```python
from build123d import *

# Parameters (mm, degrees)
SKETCH1_R                = 5.60705
BOSS_EXTRUDE1_DEPTH      = 1.778
SKETCH2_R                = 10.16
BOSS_EXTRUDE2_DEPTH      = 4.318
SKETCH3_R                = 1.143
CUT_EXTRUDE1_DEPTH       = 3.318
SKETCH4_R                = 5.5626
BOSS_EXTRUDE3_DEPTH      = 3.0099
BOSS_EXTRUDE4_DEPTH      = 5.78485
FILLET1_R                = 2
FILLET2_R                = 2
SKETCH6_W                = 8.0772
SKETCH6_H                = 4.0386
CUT_EXTRUDE2_DEPTH       = 2.6924
CHAMFER1_SIZE            = 2.6924
CHAMFER1_OF_MIRROR2_SIZE = 2.6924
FILLET3_R                = 2
BOSS_EXTRUDE5_DEPTH      = 12.7
SKETCH8_R                = 2.48285
BOSS_EXTRUDE6_DEPTH      = 25.4


with BuildPart() as part:
    # Sketch1 → Boss-Extrude1 (new body)
    with BuildSketch(Plane(origin=(0, 0, 0), x_dir=(1, 0, 0), z_dir=(0, 1, 0))):
        with Locations(Location((0, 0, 0), (0, 0, 270))):
            Circle(SKETCH1_R)
    extrude(amount=-BOSS_EXTRUDE1_DEPTH)

    # Sketch2 → Boss-Extrude2 (add)
    with BuildSketch(Plane.XZ.offset(1.778)):
        with Locations(Location((0, 0, 0), (0, 0, 270))):
            Circle(SKETCH2_R)
    extrude(amount=BOSS_EXTRUDE2_DEPTH)

    # Sketch3 → Cut-Extrude1 (cut)
    with BuildSketch(Plane(origin=(0, -1.778, 0), x_dir=(1, 0, 0), z_dir=(0, 1, 0))):
        with Locations(Location((7.4, 0, 0), (0, 0, 270))):
            Circle(SKETCH3_R)
    cut_extrude1 = extrude(amount=-CUT_EXTRUDE1_DEPTH, mode=Mode.SUBTRACT)

    # Mirror1: Cut-Extrude1 across plane
    add(cut_extrude1.mirror(Plane(origin=(0, 0, 0), x_dir=(0, 0, 1), z_dir=(1, 0, 0))), mode=Mode.SUBTRACT)

    # Sketch4 → Boss-Extrude3 (add)
    with BuildSketch(Plane.XZ.offset(6.096)):
        with Locations(Location((0, 0, 0), (0, 0, 270))):
            Circle(SKETCH4_R)
    extrude(amount=BOSS_EXTRUDE3_DEPTH)

    # Sketch5 → Boss-Extrude4 (add, symmetric)
    with BuildSketch(Plane(origin=(0, 0, 0), x_dir=(0, 0, -1), z_dir=(1, 0, 0))):
        Polygon((-8.5344, -9.1059), (8.7757, -9.1059), (8.7757, -10.0203), (11.8237, -10.0203), (11.8237, -16.51), (-5.7912, -16.51), (-11.0236, -11.7983), (-11.0236, -10.0203), (-8.5344, -10.0203), align=None)
    extrude(amount=BOSS_EXTRUDE4_DEPTH, both=True)

    # Fillet1
    fillet1_edges = [part.edges().sort_by_distance(p)[0] for p in [
        (-5.78485, -9.5631, 8.5344),
        (-5.78485, -9.5631, -8.7757),
        (5.78485, -9.5631, 8.5344),
        (5.78485, -9.5631, -8.7757),
    ]]
    fillet(fillet1_edges, radius=FILLET1_R)

    # Fillet2
    fillet2_edges = [part.edges().sort_by_distance(p)[0] for p in [
        (-5.78485, -10.9093, 11.0236),
        (5.78485, -10.9093, 11.0236),
    ]]
    fillet(fillet2_edges, radius=FILLET2_R)

    # Sketch6 → Cut-Extrude2 (cut)
    with BuildSketch(Plane(origin=(5.78485, 0, 0), x_dir=(0, 0, -1), z_dir=(1, 0, 0))):
        with Locations((7.7851, -14.4907)):
            Rectangle(SKETCH6_W, SKETCH6_H)
    cut_extrude2 = extrude(amount=-CUT_EXTRUDE2_DEPTH, mode=Mode.SUBTRACT)

    # Chamfer1
    chamfer1_edges = [part.edges().sort_by_distance(p)[0] for p in [
        (3.09245, -14.4907, -3.7465),
    ]]
    chamfer(chamfer1_edges, length=CHAMFER1_SIZE - 0.0001)  # a hair under: the kernel refuses the full size

    # Mirror2: Cut-Extrude2 across plane
    add(cut_extrude2.mirror(Plane(origin=(0, 0, 0), x_dir=(0, 0, 1), z_dir=(1, 0, 0))), mode=Mode.SUBTRACT)

    # Chamfer1 of Mirror2
    chamfer1_of_mirror2_edges = [part.edges().sort_by_distance(p)[0] for p in [
        (-3.09245, -14.4907, -3.7465),
    ]]
    chamfer(chamfer1_of_mirror2_edges, length=CHAMFER1_OF_MIRROR2_SIZE - 0.0001)  # a hair under: the kernel refuses the full size

    # Fillet3
    fillet3_edges = [part.edges().sort_by_distance(p)[0] for p in [
        (-5.78485, -11.24585, -11.8237),
        (5.78485, -11.24585, -11.8237),
    ]]
    fillet(fillet3_edges, radius=FILLET3_R)

    # Sketch7 → Boss-Extrude5 (add)
    with BuildSketch(Plane(origin=(0, 0, -11.8237), x_dir=(-1, 0, 0), z_dir=(0, 0, -1))):
        Polygon((1.529978213, -15.681103357), (3.059956427, -13.031103357), (1.529978213, -10.381103357), (-1.529978213, -10.381103357), (-3.059956427, -13.031103357), (-1.529978213, -15.681103357), align=None)
    extrude(amount=BOSS_EXTRUDE5_DEPTH)

    # Sketch8 → Boss-Extrude6 (add)
    with BuildSketch(Plane(origin=(0, 0, -24.5237), x_dir=(-1, 0, 0), z_dir=(0, 0, -1))):
        with Locations((0, -13.007748328)):
            Circle(SKETCH8_R)
    extrude(amount=BOSS_EXTRUDE6_DEPTH)


solid = part.part
```
The model under review builds one solid part; all positions refer to its coordinate system, in mm. A direction names the side the tool comes from. Round coordinates to 2 decimals unless told otherwise and drop trailing zeros. Loops run counter-clockwise (first coordinate to the right, second up) from the corner with the lowest first, then second, coordinate; pieces in that order, holes last. Notation, with made-up numbers: (1, 57.5) - (40, 57.5) arc R34 ccw to (40, 96.5) - close; hole circle Ø10 at (38, -12.5). An arc over 180 degrees is marked (long way). Use a Markdown table: item, result. Add a question column.
Q1. The part is to be moulded in two halves that separate along Y. For faces 1 (the face through (-2.306, -11.725, -18.085)), 2 (the face through (-4, -12.471, -9)), 3 (the face through (-4.4, -6.096, -4.4)), 4 (the face through (-5.215, -11.263, -11.222)), say which applies: pulls with the +Y half, pulls with the -Y half, needs draft (parallel to the pull), parting line crosses it, or undercut.
Q2. Insertion check: pin 1 Ø2.5 at (x, z) = (0.5, -21) entering from +Y; pin 2 Ø3 at (x, y) = (3.5, -5.5) entering from +Z; pin 3 Ø3 at (x, z) = (5, -30.5) entering from -Y; pin 4 Ø2.5 at (x, z) = (0.5, -9) entering from +Y. Each pin has a flat end and moves straight along its axis. Give the tip position at first contact, or say it passes through.
Q3. Add section B-B (y = -4). State the section outline as (x, z) points, plus the area to 3 significant figures.
Q4. Add section A-A (z = 0). State the section outline as (x, y) points, plus the area to 3 significant figures.
Q5. Machinability: for faces 5 (the face through (-5.785, -13, 2)), 6 (the face through (4, -12.471, -9)), 7 (the face through (0, -15.681, -18)), 8 (the face through (5.785, -13, 2)), 9 (the face through (4.73, -0.88, 3.01)), which of the approach directions +Z, -Z, +X, -X, +Y, -Y give a long, thin tool a straight path to every point of the face, cutting with its end or side? Answer none if there is none.
Q6. For probe 1 along X at (y, z) = (-3.55, 0); probe 2 along Y at (x, z) = (5.5, 5); probe 3 along Z at (x, y) = (-7.4, -4.25), list the stretches that pass through material, from the lowest coordinate up.
Q7. Add section D-D (x = -8). State the section outline as (y, z) points, plus the area to 3 significant figures.
Worked answers:
| question | item | result |
|---|---|---|
| 1 | face 1 | pulls with the +Y half |
| 1 | face 2 | pulls with the -Y half |
| 1 | face 3 | undercut |
| 1 | face 4 | needs draft |
| 2 | pin 1 | y = -10.38 |
| 2 | pin 2 | z = 9.96 |
| 2 | pin 3 | through |
| 2 | pin 4 | y = -1.78 |
| 3 | outline | circle Ø20.32 at (0, 0); hole circle Ø2.29 at (-7.4, 0); hole circle Ø2.29 at (7.4, 0) |
| 3 | area | 316 mm² |
| 4 | outline | (-10.16, -6.1) - (-5.56, -6.1) - (-5.56, -9.11) - (-5.78, -9.11) - (-5.78, -16.51) - (5.78, -16.51) - (5.78, -9.11) - (5.56, -9.11) - (5.56, -6.1) - (10.16, -6.1) - (10.16, -1.78) - (8.54, -1.78) - (8.54, -5.1) - (6.26, -5.1) - (6.26, -1.78) - (5.61, -1.78) - (5.61, 0) - (-5.61, 0) - (-5.61, -1.78) - (-6.26, -1.78) - (-6.26, -5.1) - (-8.54, -5.1) - (-8.54, -1.78) - (-10.16, -1.78) - close |
| 4 | area | 212 mm² |
| 5 | face 5 | +Z, -Z, -X, -Y |
| 5 | face 6 | -Z, +X, -Y |
| 5 | face 7 | -Z, +X, -X, -Y |
| 5 | face 8 | +Z, -Z, +X, -Y |
| 5 | face 9 | +Y |
| 6 | probe 1 | -10.16 to -8.54, -6.26 to 6.26, 8.54 to 10.16 |
| 6 | probe 2 | -16.51 to -9.11, -6.1 to -1.78 |
| 6 | probe 3 | -6.96 to -1.14, 1.14 to 6.96 |
| 7 | outline | (-6.1, -6.26) - (-1.78, -6.26) - (-1.78, -0.97) - (-5.1, -0.97) - (-5.1, 0.97) - (-1.78, 0.97) - (-1.78, 6.26) - (-6.1, 6.26) - close |
| 7 | area | 47.6 mm² |
